Work out the finished part from the listing and answer in its coordinate system (mm). Face numbers are marked on the shaded views. A direction names the side the tool comes from. Give positions to 0.01 mm unless a question says otherwise; leave off trailing zeros. Order: outer loops, then holes, each group sorted by start corner. A loop starts at its lowest first (then second) coordinate and runs counter-clockwise, first axis right, second up. Notation, with made-up numbers: (10, 41) - (20, 41) arc R32 ccw to (20, 75) - close; hole circle Ø1 at (25, 10). An arc over 180 degrees is marked (long way). Write each question's results on one line, items separated by ' | '.
from build123d import *

# Parameters (mm, degrees)
SKETCH_1_W      = 46
SKETCH_1_H      = 32
EXTRUDE_1_DEPTH = 22
SKETCH_2_R      = 12
EXTRUDE_2_DEPTH = 31
SKETCH_3_R      = 5
EXTRUDE_3_DEPTH = 1
SKETCH_4_R      = 3
EXTRUDE_4_DEPTH = 14
SKETCH_5_R      = 3.5
EXTRUDE_5_DEPTH = 1


with BuildPart() as part:
    # Эскиз1 → Бобышка-Вытянуть1 (new body)
    with BuildSketch(Plane(origin=(0, 0, 0), x_dir=(1, 0, 0), z_dir=(0, 1, 0))):
        Rectangle(SKETCH_1_W, SKETCH_1_H)
    extrude(amount=EXTRUDE_1_DEPTH)

    # Эскиз2 → Бобышка-Вытянуть2 (add)
    with BuildSketch(Plane(origin=(23, 0, 0), x_dir=(0, 0, -1), z_dir=(1, 0, 0))):
        with Locations(Location((0, 10, 0), (0, 0, 236.442690238))):
            Circle(SKETCH_2_R)
    extrude(amount=EXTRUDE_2_DEPTH)

    # Эскиз3 → Бобышка-Вытянуть3 (add)
    with BuildSketch(Plane(origin=(0, 22, 0), x_dir=(1, 0, 0), z_dir=(0, 1, 0))):
        with Locations(Location((-11.5, 0, 0), (0, 0, 90))):
            Circle(SKETCH_3_R)
    extrude(amount=EXTRUDE_3_DEPTH)

    # Эскиз4 → Бобышка-Вытянуть4 (add)
    with BuildSketch(Plane(origin=(0, 23, 0), x_dir=(1, 0, 0), z_dir=(0, 1, 0))):
        with Locations(Location((-11.5, 0, 0), (0, 0, 270))):
            Circle(SKETCH_4_R)
    extrude(amount=EXTRUDE_4_DEPTH)

    # Эскиз5 → Бобышка-Вытянуть5 (add)
    with BuildSketch(Plane(origin=(0, 22, 0), x_dir=(1, 0, 0), z_dir=(0, 1, 0))):
        with Locations(Location((18, 11, 0), (0, 0, 90))):
            Circle(SKETCH_5_R)
        with Locations(Location((18, -11, 0), (0, 0, 90))):
            Circle(SKETCH_5_R)
        with Locations(Location((-18, -11, 0), (0, 0, 90))):
            Circle(SKETCH_5_R)
        with Locations(Location((-18, 11, 0), (0, 0, 90))):
            Circle(SKETCH_5_R)
    extrude(amount=EXTRUDE_5_DEPTH)


solid = part.part
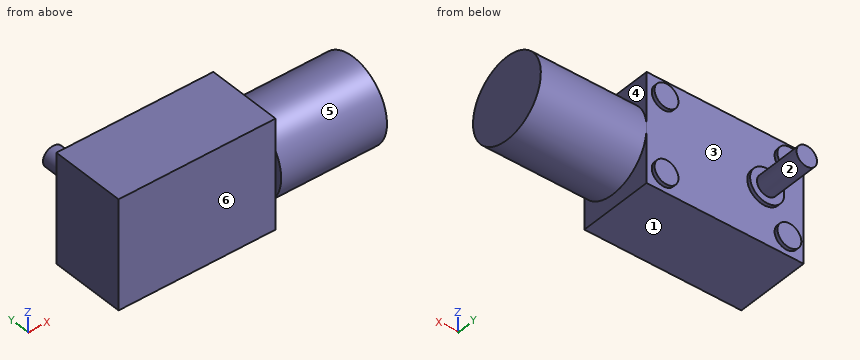
1. A cutting plane is placed at A-A, the plane x = 18. Write down the section's boundary in (y, z).
Answer list:
outline: (0, -16) - (22, -16) - (22, -14.5) - (23, -14.5) - (23, -7.5) - (22, -7.5) - (22, 7.5) - (23, 7.5) - (23, 14.5) - (22, 14.5) - (22, 16) - (0, 16) - close
2. A cutting plane is placed at C-C, the plane z = -9.5. Write down the section's boundary in (x, y), then the cut area to 3 significant figures.
Answer list:
outline: (-23, 0) - (23, 0) - (23, 2.67) - (54, 2.67) - (54, 17.33) - (23, 17.33) - (23, 22) - (21.16, 22) - (21.16, 23) - (14.84, 23) - (14.84, 22) - (-14.84, 22) - (-14.84, 23) - (-21.16, 23) - (-21.16, 22) - (-23, 22) - close | area: 1,480 mm^2
3. A cutting plane is placed at D-D, the plane x = -15.5. Write down the section's boundary in (y, z).
Answer list:
outline: (0, -16) - (22, -16) - (22, -13.45) - (23, -13.45) - (23, -8.55) - (22, -8.55) - (22, -3) - (23, -3) - (23, 3) - (22, 3) - (22, 8.55) - (23, 8.55) - (23, 13.45) - (22, 13.45) - (22, 16) - (0, 16) - close
4. Straight lines are drawn through the part: line 1 (X direction, y = 1, z = 11.5); line 2 (Y direction, x = -3.5, z = -7); line 3 (Y direction, x = -9.5, z = -2.5). For each, find the intervals that lie inside material, in ascending order. Write a range as [from, to].
Answer list:
line 1: [-23, 23] | line 2: [0, 22] | line 3: [0, 23]
5. Determine the mould class of the marked faces 1, 2 and 3 for opening direction X: +X half, -X half, draft (parallel to the pull), parting line (faces both ways), or undercut.
Answer list:
face 1: draft | face 2: parting line | face 3: undercut
6. Given P1, Ø2, axis at x = 42.5, z = 9, coming from the +Y side; P2, Ø1.6, axis at y = -1.5, z = -2.5, coming from the -X side; P3, Ø5.5, axis at x = -19.5, z = 11, coming from the +Y side; P4, Ø5, axis at y = 25.5, z = 7, coming from the -X side, each flat-ended and moving along its own axis, determine where each tip first touches the part or whether it passes through.
Answer list:
P1: y = 18.94 | P2: x = 23 | P3: y = 23 | P4: through
7. A tool of negligible diameter and unlimited length cuts with its end or side. For the marked faces 4, 5 and 6, from which of +Z, -Z, +X, -X, +Y, -Y can it reach the whole face along a straight path? Write none if from no direction.
Answer list:
face 4: +Z, +X | face 5: +X | face 6: +Z, -Z, -X, -Y
8. A cutting plane is placed at B-B, the plane y = 10. Write down the section's boundary in (x, z).
Answer list:
outline: (-23, -16) - (23, -16) - (23, -12) - (54, -12) - (54, 12) - (23, 12) - (23, 16) - (-23, 16) - close
